For this review, take the finished solid that the model builds, in its own axes (mm). A direction names the side the tool comes from. Give positions to 0.01 mm unless a question says otherwise; leave off trailing zeros. Order: outer loops, then holes, each group sorted by start corner. A loop starts at its lowest first (then second) coordinate and runs counter-clockwise, first axis right, second up. Notation, with made-up numbers: (71.5, -27) - (89.5, -27) arc R25 ccw to (89.5, -15) - close; hole circle Ø7 at (-22.5, 5.5). An arc over 180 degrees is marked (long way). One line per item, written item: value.
```python
from build123d import *

# Parameters (mm, degrees)
BOSS_EXTRUDE1_DEPTH = 15
BOSS_EXTRUDE2_DEPTH = 10


with BuildPart() as part:
    # Sketch3 → Boss-Extrude1 (new body)
    with BuildSketch(Plane.XY):
        with BuildLine():
            Line((230, 20), (230, -20))
            Line((230, -20), (30, -20))
            ThreePointArc((30, -20), (36.055512755, 0), (30, 20))
            Line((30, 20), (230, 20))
        make_face()
    extrude(amount=-BOSS_EXTRUDE1_DEPTH)

    # Sketch6 → Boss-Extrude2 (add)
    with BuildSketch(Plane(origin=(0, 0, -15), x_dir=(-1, 0, 0), z_dir=(0, 0, -1))):
        with BuildLine():
            Line((-37.273180707, 20), (-30, 20))
            ThreePointArc((-30, 20), (-36.055512755, 0), (-30, -20))
            Line((-30, -20), (-37.273180707, -20))
            ThreePointArc((-37.273180707, -20), (-42.3, 0), (-37.273180707, 20))
        make_face()
        with BuildLine():
            Line((-46.043892103, 20), (-58.043892103, 20))
            ThreePointArc((-58.043892103, 20), (-61.392942676, 0), (-58.043892103, -20))
            Line((-58.043892103, -20), (-46.043892103, -20))
            ThreePointArc((-46.043892103, -20), (-50.2, 0), (-46.043892103, 20))
        make_face()
    extrude(amount=BOSS_EXTRUDE2_DEPTH)


solid = part.part
```
(1) Take a section at A-A (z = -18.75). Write out the cut boundary in (x, y), then the cut area to 3 significant figures.
Answers below:
outline: (30, -20) - (37.27, -20) arc R42.3 ccw to (37.27, 20) - (30, 20) arc R36.06 cw to start; (46.04, -20) - (58.04, -20) arc R61.39 ccw to (58.04, 20) - (46.04, 20) arc R50.2 cw to start
area: 720 mm^2
(2) Machinability: for faces 5 (the face through (61.392, 0.285, -19.93)), 6 (the face through (42.3, -0.3, -19.9)), 7 (the face through (131, 0, 0)), which of the approach directions +Z, -Z, +X, -X, +Y, -Y give a long, thin tool a straight path to every point of the face, cutting with its end or side? Answer none if there is none.
Answers below:
face 5: -Z, +X
face 6: -Z
face 7: +Z, +X, -X, +Y, -Y
(3) Draft analysis for pull direction Y (two halves, no side actions). For faces 1 (the face through (45, 0, -15)), 2 (the face through (131, 20, -7)), 3 (the face through (230, 0, -7)), 4 (the face through (129, -20, -7)), state which applies: pulls with the +Y half, pulls with the -Y half, needs draft (parallel to the pull), parting line crosses it, or undercut.
Answers below:
face 1: undercut
face 2: pulls with the +Y half
face 3: needs draft
face 4: pulls with the -Y half
(4) Take a section at B-B (y = -14.5). Write out the cut boundary in (x, z).
Answers below:
outline: (33.01, -25) - (39.74, -25) - (39.74, -15) - (48.06, -15) - (48.06, -25) - (59.66, -25) - (59.66, -15) - (230, -15) - (230, 0) - (33.01, 0) - close
(5) Take a section at C-C (x = 82.5). Write out the cut boundary in (y, z), then the cut area to 3 significant figures.
Answers below:
outline: (-20, -15) - (20, -15) - (20, 0) - (-20, 0) - close
area: 600 mm^2
(6) For P1, Ø10, axis at x = 198, y = 15, coming from the -Z side; P2, Ø5, axis at y = 14, z = -19, coming from the +X side, all flat-tipped, find the tip position at first contact; note any pin that passes through.
Answers below:
P1: stops at z = -15
P2: stops at x = 60.31
(7) Wall thickness on line 1 (Z direction, x = 45, y = -6.5); line 2 (X direction, y = -5.5, z = -15.5); line 3 (X direction, y = 13, z = -20): over which ranges is each line inside the solid? List them lowest first. Write a range as from..to.
Answers below:
line 1: z = -15..0
line 2: x = 35.63..41.94, 49.9..61.15
line 3: x = 33.63..40.25, 48.49..60
(8) Take a section at D-D (z = -11.25). Write out the cut boundary in (x, y).
Answers below:
outline: (30, -20) - (230, -20) - (230, 20) - (30, 20) arc R36.06 cw to start
